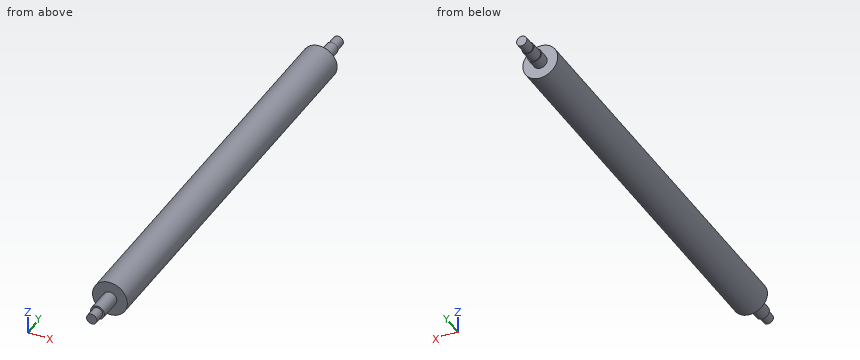
```python
from build123d import *

# Parameters (mm, degrees)
SKETCH1_R            = 10
BOSS_EXTRUDE8_DEPTH  = 236
SKETCH1_9_R          = 3.965
BOSS_EXTRUDE9_DEPTH  = 14
BOSS_EXTRUDE10_START = -14
SKETCH1_10_R         = 2.95
BOSS_EXTRUDE10_DEPTH = 6.5
BOSS_EXTRUDE11_START = 242.5
SKETCH1_11_R         = 3.965
BOSS_EXTRUDE11_DEPTH = 6.5
BOSS_EXTRUDE12_START = 242.5
SKETCH1_12_R         = 3.45
BOSS_EXTRUDE12_DEPTH = 7.3
BOSS_EXTRUDE13_START = 256.9
SKETCH1_13_R         = 2.95
BOSS_EXTRUDE13_DEPTH = 7.1


with BuildPart() as part:
    # Sketch1 → Boss-Extrude8 (new body)
    with BuildSketch(Plane(origin=(0, 0, 0), x_dir=(1, 0, 0), z_dir=(0, 1, 0))):
        with Locations(Location((0, 0, 0), (0, 0, 270))):
            Circle(SKETCH1_R)
    extrude(amount=BOSS_EXTRUDE8_DEPTH)

    # Sketch1<9> → Boss-Extrude9 (add)
    with BuildSketch(Plane(origin=(0, 0, 0), x_dir=(1, 0, 0), z_dir=(0, 1, 0))):
        with Locations(Location((0, 0, 0), (0, 0, 270))):
            Circle(SKETCH1_9_R)
    extrude(amount=-BOSS_EXTRUDE9_DEPTH)

    # Sketch1<10> → Boss-Extrude10 (add)
    with BuildSketch(Plane(origin=(0, 0, 0), x_dir=(1, 0, 0), z_dir=(0, 1, 0)).offset(BOSS_EXTRUDE10_START)):
        with Locations(Location((0, 0, 0), (0, 0, 270))):
            Circle(SKETCH1_10_R)
    extrude(amount=-BOSS_EXTRUDE10_DEPTH)

    # Sketch1<11> → Boss-Extrude11 (add)
    with BuildSketch(Plane(origin=(0, 0, 0), x_dir=(1, 0, 0), z_dir=(0, 1, 0)).offset(BOSS_EXTRUDE11_START)):
        with Locations(Location((0, 0, 0), (0, 0, 270))):
            Circle(SKETCH1_11_R)
    extrude(amount=-BOSS_EXTRUDE11_DEPTH)

    # Sketch1<12> → Boss-Extrude12 (add)
    with BuildSketch(Plane(origin=(0, 0, 0), x_dir=(1, 0, 0), z_dir=(0, 1, 0)).offset(BOSS_EXTRUDE12_START)):
        with Locations(Location((0, 0, 0), (0, 0, 270))):
            Circle(SKETCH1_12_R)
    extrude(amount=BOSS_EXTRUDE12_DEPTH)

    # Sketch1<13> → Boss-Extrude13 (add)
    with BuildSketch(Plane(origin=(0, 0, 0), x_dir=(1, 0, 0), z_dir=(0, 1, 0)).offset(BOSS_EXTRUDE13_START)):
        with Locations(Location((0, 0, 0), (0, 0, 270))):
            Circle(SKETCH1_13_R)
    extrude(amount=-BOSS_EXTRUDE13_DEPTH)


solid = part.part
```
Design review of the part built by this model. Coordinates are the model's own, in mm. Give positions to 0.01 mm unless a question says otherwise; leave off trailing zeros. Write each loop counter-clockwise with the first axis right and the second up, starting at its lowest first coordinate (ties: lowest second). Pieces come first, ordered by that corner, then holes. Notation, with made-up numbers: (-15, -23.5) - (0, -23.5) arc R22 ccw to (0, -11.5) - close; hole circle Ø8 at (-6, -9.75). An arc over 180 degrees is marked (long way). Return JSON: item names as keys, results as strings. Group by question number.
(1) We need section C-C, the plane y = 71.5. Give the boundary of the cut face in (x, z), then the cut area to 3 significant figures.
(2) To check wall thickness, follow probe 1 along Y at (x, z) = (8.25, -5.25); probe 2 along Z at (x, y) = (0.75, 115.5); probe 3 along X at (y, z) = (237.5, -0.5). State the ranges of each line that lie inside material, in increasing order.
(3) Insertion check: pin 1 (1 mm diameter, centred on x = -5.5, y = 187.5, fed in from +Z); pin 2 (1 mm diameter, centred on y = 45, z = 1, fed in from +X); pin 3 (6 mm diameter, centred on x = -5, y = 133, fed in from -Z). Each pin has a flat end and moves straight along its axis. Give the tip position at first contact, or say it passes through.
(4) We need section A-A, the plane x = 0. Give the boundary of the cut face in (y, z) (3 decimals), then the cut area to 3 significant figures.
(5) We need section B-B, the plane z = 0. Give the boundary of the cut face in (x, y) (3 decimals).
Reported:
{
 "1": {"outline": "circle Ø20 at (0, 0)", "area": "314 mm2"},
 "2": {"probe 1": "y = 0 to 236", "probe 2": "z = -9.97 to 9.97", "probe 3": "x = -3.93 to 3.93"},
 "3": {"pin 1": "stops at z = 8.66", "pin 2": "stops at x = 9.99", "pin 3": "stops at z = -9.8"},
 "4": {"outline": "(-20.5, -2.95) - (-14, -2.95) - (-14, -3.965) - (0, -3.965) - (0, -10) - (236, -10) - (236, -3.965) - (242.5, -3.965) - (242.5, -3.45) - (249.8, -3.45) - (249.8, -2.95) - (256.9, -2.95) - (256.9, 2.95) - (249.8, 2.95) - (249.8, 3.45) - (242.5, 3.45) - (242.5, 3.965) - (236, 3.965) - (236, 10) - (0, 10) - (0, 3.965) - (-14, 3.965) - (-14, 2.95) - (-20.5, 2.95) - close", "area": "5,010 mm2"},
 "5": {"outline": "(-10, 0) - (-3.965, 0) - (-3.965, -14) - (-2.95, -14) - (-2.95, -20.5) - (2.95, -20.5) - (2.95, -14) - (3.965, -14) - (3.965, 0) - (10, 0) - (10, 236) - (3.965, 236) - (3.965, 242.5) - (3.45, 242.5) - (3.45, 249.8) - (2.95, 249.8) - (2.95, 256.9) - (-2.95, 256.9) - (-2.95, 249.8) - (-3.45, 249.8) - (-3.45, 242.5) - (-3.965, 242.5) - (-3.965, 236) - (-10, 236) - close"}
}
